Work out the finished part from the listing and answer in its coordinate system (mm). A direction names the side the tool comes from. Round coordinates to 2 decimals unless told otherwise and drop trailing zeros. Order: outer loops, then holes, each group sorted by start corner. A loop starts at its lowest first (then second) coordinate and runs counter-clockwise, first axis right, second up. Notation, with made-up numbers: (-24.5, -34.75) - (18.5, -34.75) arc R29 ccw to (18.5, 2.25) - close; hole circle Ø3 at (63, 79). An arc over 180 degrees is marked (long way). Use one line per item in the form item = value. Start each with the question number.
Q1. The part is cut by section A-A on x = -16.28. Determine the outline of the cut face in (y, z) (3 decimals), plus the area to 3 significant figures.
Q2. Given P1, Ø5, axis at y = 23, z = 7.5, coming from the +X side; P2, Ø1.5, axis at y = -3, z = 2.5, coming from the +X side; P3, Ø3, axis at y = 26.5, z = 5.5, coming from the -X side; P4, Ø12, axis at x = 4, y = 8.5, coming from the +Z side, each flat-ended and moving along its own axis, determine where each tip first touches the part or whether it passes through.
Q3. Which of the six approach directions +Z, -Z, +X, -X, +Y, -Y give full straight-line access (tool end or side, diameter ignored) to faces 1 (the flat face through (5.17, 25, 6)), 2 (the flat face through (-1, 17, 6)), 3 (the flat face through (-1, 29, 1))?
Q4. Find the intervals of material crossed by line 1 (Y direction, x = -16.28, z = 0.6) (3 decimals); line 2 (Z direction, x = 12, y = -18.5); line 3 (X direction, y = 22, z = 9.75), in increasing order. Write a range as [from, to].
Q5. The part is cut by section B-B on y = -21.28. Determine the outline of the cut face in (x, z) (3 decimals), plus the area to 3 significant figures.
Q6. The part is cut by section C-C on z = 8. Determine the outline of the cut face in (x, y).
Q7. The part is cut by section D-D on y = 21.28. Determine the outline of the cut face in (x, z) (3 decimals).
from build123d import *

# Parameters (mm, degrees)
F0_W     = 40
F0_H     = 50
F0_R     = 1.695
F1_DEPTH = 1
F2_W     = 12
F2_H     = 16
F3_DEPTH = 10


with BuildPart() as f1:
    # F0 (on Top) → F1 (new body)
    with BuildSketch(Plane.XY):
        Rectangle(F0_W, F0_H)
        with Locations((-16.28, -21.28)):
            Circle(F0_R, mode=Mode.SUBTRACT)
        with Locations((16.28, -21.28)):
            Circle(F0_R, mode=Mode.SUBTRACT)
        with Locations((-16.28, 21.28)):
            Circle(F0_R, mode=Mode.SUBTRACT)
        with Locations((16.28, 21.28)):
            Circle(F0_R, mode=Mode.SUBTRACT)
    extrude(amount=F1_DEPTH)

    # F2 (on face) → F3 (join)
    with BuildSketch(Plane.XY.offset(1)):
        with Locations((-0.82982, 25)):
            Rectangle(F2_W, F2_H)
    extrude(amount=F3_DEPTH)


solid = f1.part
Found:
q1.outline = (-25, 0) - (-22.975, 0) - (-22.975, 1) - (-25, 1) - close; (-19.585, 0) - (19.585, 0) - (19.585, 1) - (-19.585, 1) - close; (22.975, 0) - (25, 0) - (25, 1) - (22.975, 1) - close
q1.area = 43.2 mm²
q2.P1 = 5.17
q2.P2 = through
q2.P3 = -6.83
q2.P4 = 1
q3.face_1 = +Z, +X, +Y, -Y
q3.face_2 = +Z, +X, -X, -Y
q3.face_3 = -Z, +X, -X, +Y
q4.line_1 = [-25, -22.975], [-19.585, 19.585], [22.975, 25]
q4.line_2 = [0, 1]
q4.line_3 = [-6.83, 5.17]
q5.outline = (-20, 0) - (-17.975, 0) - (-17.975, 1) - (-20, 1) - close; (-14.585, 0) - (14.585, 0) - (14.585, 1) - (-14.585, 1) - close; (17.975, 0) - (20, 0) - (20, 1) - (17.975, 1) - close
q5.area = 33.2 mm²
q6.outline = (-6.83, 17) - (5.17, 17) - (5.17, 33) - (-6.83, 33) - close
q7.outline = (-20, 0) - (-17.975, 0) - (-17.975, 1) - (-20, 1) - close; (-14.585, 0) - (14.585, 0) - (14.585, 1) - (5.17, 1) - (5.17, 11) - (-6.83, 11) - (-6.83, 1) - (-14.585, 1) - close; (17.975, 0) - (20, 0) - (20, 1) - (17.975, 1) - close
